```python
from build123d import *

# Parameters (mm, degrees)
F0_W      = 9.525
F0_H      = 4.380480709
F1_DEPTH  = 1.27
F2_W      = 2.9321946495
F2_H      = 12.622077018
F3_DEPTH  = 2.54
F6_DEPTH  = 25.4
F8_DEPTH  = 25.4
F9_R      = 0.9600996903
F10_DEPTH = 25.4
F11_W     = 2.0492244512
F11_H     = 10.8852496778
F12_DEPTH = 2.286
F13_W     = 10.9546062886
F13_H     = 1.8707374111
F14_DEPTH = 25.4


with BuildPart() as f1:
    # F0 (on Top) → F1 (new body)
    with BuildSketch(Plane.XY):
        with Locations((-23.2204422355, 6.7132576369)):
            Rectangle(F0_W, F0_H)
    extrude(amount=F1_DEPTH)

    # F2 (on face) → F3 (join)
    with BuildSketch(Plane.XY.offset(1.27)):
        with Locations((-23.2204422355, 6.311038509)):
            Rectangle(F2_W, F2_H)
    extrude(amount=F3_DEPTH)

    # F5 (on face) → F6 (cut)
    with BuildSketch(Plane.YZ.offset(-18.4579422355)):
        Polygon((4.5230172824, 1.27), (4.5230172824, 0), (5.1185246557, 1.27), align=None)
        Polygon((8.3203641698, 1.27), (8.9034979914, 0), (8.9034979914, 1.27), align=None)
    extrude(amount=-F6_DEPTH, mode=Mode.SUBTRACT)

    # F7 (on face) → F8 (cut)
    with BuildSketch(Plane.YZ.offset(-21.7543449107)):
        Polygon((11.8150692433, 3.81), (12.622077018, 1.27), (12.622077018, 3.81), align=None)
    extrude(amount=-F8_DEPTH, mode=Mode.SUBTRACT)

    # F9 (on face) → F10 (cut)
    with BuildSketch(Plane.XZ):
        with Locations((-23.2783449107, 2.6081991382)):
            Circle(F9_R)
    extrude(amount=-F10_DEPTH, mode=Mode.SUBTRACT)

    # F11 (on face) → F12 (cut)
    with BuildSketch(Plane.XY.offset(3.81)):
        with Locations((-23.2297061011, 5.8172373829)):
            Rectangle(F11_W, F11_H)
    extrude(amount=-F12_DEPTH, mode=Mode.SUBTRACT)

    # F13 (on face) → F14 (cut)
    with BuildSketch(Plane.YZ.offset(-21.7543449107)):
        with Locations((6.1044846952, 2.4918210693)):
            Rectangle(F13_W, F13_H)
    extrude(amount=-F14_DEPTH, mode=Mode.SUBTRACT)


solid = f1.part
```
Geometry: final body of the model. Coordinates: model frame, mm. A direction names the side the tool comes from. Coordinates: 2 decimals unless noted, no trailing zeros. Order: outer loops, then holes, each group sorted by start corner. A loop starts at its lowest first (then second) coordinate and runs counter-clockwise, first axis right, second up. Notation, with made-up numbers: M 38.25,75.5 L 59.25,75.5 A10 cw 59.25,88.5 Z; hole C 72.5,73 d9. An arc over 180 degrees is marked long. Answer in a Markdown table with one row per item. Add a question column.
Q1. Contact query for flat-ended pins moving along their axis: P1, Ø2, axis at y = 3.5, z = 2, coming from the -X side; P2, Ø1, axis at x = -24, y = 7, coming from the -Z side; P3, Ø2, axis at y = 3.5, z = 2.5, coming from the +X side; P4, Ø1.5, axis at x = -23.28, z = 2.61, coming from the -Y side. Output: stop coordinate, or through.
Q2. Section query A-A on y = 7.75. Count the separate pieces of the cut face and the enclosed holes in it, and give its area (3 significant figures).
Q3. Section query D-D on x = -19.5. Return the cut outline in (y, z).
Q4. Line query: L1, parallel to Z at x = -24.5, y = 3; L2, parallel to Z at x = -22.25, y = 10.75; L3, parallel to Y at x = -22.25, z = 2.1. Output: solid intervals per line, ascending.
Q5. Mould query, pull axis X, two halves, no side actions, for faces 6 (the flat face through (-24.687, 6.22, 3.65)), 7 (the flat face through (-18.458, 7, 1)), 8 (the cylindrical face through (-22.39, 0.18, 2.24)). Classes: released by +X, released by -X, zero draft, split by the parting line, or undercut.
Q6. Reachability of faces 1 (the flat face through (-20, 7, 1.27)), 2 (the flat face through (-26, 7, 1.27)), 3 (the flat face through (-23.15, 4.82, 0.63)), 4 (the flat face through (-22.205, 5.4, 3.6)), 5 (the flat face through (-22, 6, 1.556)) from +Z, -Z, +X, -X, +Y, -Y: full face, straight path, thin tool, end or side. Return the list, or none.
Completed:
| question | item | result |
|---|---|---|
| 1 | P1 | stops at x = -24.69 |
| 1 | P2 | stops at z = 0 |
| 1 | P3 | stops at x = -21.75 |
| 1 | P4 | passes through |
| 2 | separate pieces | 3 |
| 2 | enclosed holes | 0 |
| 2 | area | 13.2 mm2 |
| 3 | outline | M 4.52,0 L 8.9,0 L 8.32,1.27 L 5.12,1.27 Z |
| 4 | L1 | z = 1.27 to 1.56, 3.43 to 3.81 |
| 4 | L2 | z = 1.27 to 1.52 |
| 4 | L3 | y = 0 to 0.37, 11.58 to 12.36 |
| 5 | face 6 | released by -X |
| 5 | face 7 | released by +X |
| 5 | face 8 | undercut |
| 6 | face 1 | +Z, +X, +Y, -Y |
| 6 | face 2 | +Z, -X, +Y, -Y |
| 6 | face 3 | +X, -X, -Y |
| 6 | face 4 | +Z |
| 6 | face 5 | +X, -X |
